Design review of the part built by this model. Coordinates are the model's own, in mm. A direction names the side the tool comes from. Give positions to 0.01 mm unless a question says otherwise; leave off trailing zeros. Answer in a Markdown table with one row per item. Add a question column.
(1) For line 1 (Z direction, x = 0, y = 0.8) (1 decimal); line 2 (X direction, y = 1.85, z = 0) (1 decimal); line 3 (Z direction, x = 6.75, y = 2), list the stretches that pass through material, from the lowest coordinate up.
(2) Draft analysis for pull direction Z (two halves, no side actions). For faces 1 (the cylindrical face through (14.28, 1.57, -0.49)), 2 (the flat face through (-8, 2, -7.938)), 3 (the flat face through (10, 3.175, -1)), state which applies: +Z half, -Z half, draft (parallel to the pull), parting line (faces both ways), or undercut.
(3) For faces 4 (the flat face through (-8, 2, 7.938)), 5 (the cylindrical face through (9.52, 1.57, 0.28)), list the 3-axis set-ups (+Z, -Z, +X, -X, +Y, -Y) from which the entire face can be reached by the end or side of a thin tool; tool diameter is ignored.
(4) For pin 1 (1.5 mm diameter, centred on y = 2.5, z = 5.5, fed in from -X); pin 2 (1.3 mm diameter, centred on x = -7, y = 2, fed in from -Z); pin 3 (1 mm diameter, centred on y = 0.5, z = -4.5, fed in from +X); pin 4 (15 mm diameter, centred on x = 0, z = 0, fed in from -Y), all flat-tipped, find the tip position at first contact; note any pin that passes through.
from build123d import *

# Parameters (mm, degrees)
F1_DEPTH = 3.175
F2_SIZE  = 0.254


with BuildPart() as f1:
    # F0 (on Front) → F1 (new body)
    with BuildSketch(Plane.XZ):
        with BuildLine():
            ThreePointArc((-10.246941, -7.9375), (-10.985066, -8.409984), (-10.865041, -9.278122))
            ThreePointArc((-10.865041, -9.278122), (14.2875, 0), (-10.865041, 9.278122))
            ThreePointArc((-10.865041, 9.278122), (-10.985066, 8.409984), (-10.246941, 7.9375))
            Line((-10.246941, 7.9375), (-5.504758, 7.9375))
            ThreePointArc((-5.504758, 7.9375), (-5.279535, 7.969327), (-5.071951, 8.062316))
            ThreePointArc((-5.071951, 8.062316), (9.525, 0), (-5.071951, -8.062316))
            ThreePointArc((-5.071951, -8.062316), (-5.279535, -7.969327), (-5.504758, -7.9375))
            Line((-5.504758, -7.9375), (-10.246941, -7.9375))
        make_face()
    extrude(amount=-F1_DEPTH)

    # F2
    f2_edges = [f1.edges().sort_by_distance(p)[0] for p in [
        (9.525, 0, 0),
        (9.525, 3.175, 0),
    ]]
    chamfer(f2_edges, length=F2_SIZE)


solid = f1.part
Values follow:
| question | item | result |
|---|---|---|
| 1 | line 1 | -14.3 to -9.5, 9.5 to 14.3 |
| 1 | line 2 | 9.5 to 14.3 |
| 1 | line 3 | -12.59 to -6.72, 6.72 to 12.59 |
| 2 | face 1 | parting line |
| 2 | face 2 | undercut |
| 2 | face 3 | draft |
| 3 | face 4 | -X, +Y, -Y |
| 3 | face 5 | +Y, -Y |
| 4 | pin 1 | x = 7.19 |
| 4 | pin 2 | z = -12.8 |
| 4 | pin 3 | x = 13.72 |
| 4 | pin 4 | through |
